For this review, take the finished solid that the model builds, in its own axes (mm). A direction names the side the tool comes from. Give positions to 0.01 mm unless a question says otherwise; leave off trailing zeros. Write each loop counter-clockwise with the first axis right and the second up, starting at its lowest first coordinate (ties: lowest second). Pieces come first, ordered by that corner, then holes. Notation, with made-up numbers: (53.5, 2.5) -> (60.5, 2.5) arc R11 ccw to (60.5, 9.5) -> close; hole circle Ø5 at (67, 31). An arc over 180 degrees is marked (long way). Answer as CSV lines item,"result".
```python
from build123d import *

# Parameters (mm, degrees)
F0_W     = 60
F0_H     = 40
F0_R     = 1
F1_DEPTH = 2
F2_W     = 8.5
F2_H     = 19
F3_DEPTH = 4
F4_W     = 34
F4_H     = 19
F5_DEPTH = 7
F6_W     = 2.5
F6_H     = 15
F6_W_2   = 6.5
F7_DEPTH = 4.3


with BuildPart() as f1:
    # F0 (on Front) → F1 (new body)
    with BuildSketch(Plane.XZ):
        Rectangle(F0_W, F0_H)
        with Locations((-28, -18)):
            Circle(F0_R, mode=Mode.SUBTRACT)
        with Locations((28, -18)):
            Circle(F0_R, mode=Mode.SUBTRACT)
        with Locations((-28, 18)):
            Circle(F0_R, mode=Mode.SUBTRACT)
        with Locations((28, 18)):
            Circle(F0_R, mode=Mode.SUBTRACT)
    extrude(amount=F1_DEPTH)

    # F2 (on face) → F3 (join)
    with BuildSketch(Plane(origin=(0, 0, 0), x_dir=(-1, 0, 0), z_dir=(0, 1, 0))):
        with Locations((20.25, 4.5)):
            Rectangle(F2_W, F2_H)
    extrude(amount=F3_DEPTH)

    # F4 (on face) → F5 (join)
    with BuildSketch(Plane(origin=(0, 0, 0), x_dir=(-1, 0, 0), z_dir=(0, 1, 0))):
        with Locations((-6.5, 3.5)):
            Rectangle(F4_W, F4_H)
    extrude(amount=F5_DEPTH)

    # F6 (on face) → F7 (join)
    with BuildSketch(Plane(origin=(0, 7, 0), x_dir=(-1, 0, 0), z_dir=(0, 1, 0))):
        with Locations((-22.25, 3.5)):
            Rectangle(F6_W, F6_H)
        with Locations((-26.75, 3.5)):
            Rectangle(F6_W_2, F6_H)
    extrude(amount=F7_DEPTH)


solid = f1.part
```
Q1. Add section C-C (z = 18). Write out the cut boundary in (x, y).
Answer block:
outline,"(-30, -2) -> (-29, -2) -> (-29, 0) -> (-30, 0) -> close; (-27, -2) -> (27, -2) -> (27, 0) -> (-27, 0) -> close; (29, -2) -> (30, -2) -> (30, 0) -> (29, 0) -> close"
Q2. Add section A-A (x = 28). Write out the cut boundary in (y, z).
Answer block:
outline,"(-2, -20) -> (0, -20) -> (0, -19) -> (-2, -19) -> close; (-2, -17) -> (0, -17) -> (0, 17) -> (-2, 17) -> close; (-2, 19) -> (0, 19) -> (0, 20) -> (-2, 20) -> close; (7, -4) -> (11.3, -4) -> (11.3, 11) -> (7, 11) -> close"
Q3. Clearance check with flat-ended pins moving along their axes: pin 1 (3.5 mm diameter, centred on x = 7.5, y = 2.5, fed in from +Z); pin 2 (4.5 mm diameter, centred on x = 27.5, y = 9.5, fed in from -Z); pin 3 (2.5 mm diameter, centred on x = 28, z = -18, fed in from +Y). State where each tip first meets the part, or that it passes through.
Answer block:
pin 1,"stops at z = 13"
pin 2,"stops at z = -4"
pin 3,"stops at y = 0"
Q4. Add section D-D (x = -5.5). Write out the cut boundary in (y, z), plus the area to 3 significant figures.
Answer block:
outline,"(-2, -20) -> (0, -20) -> (0, -6) -> (7, -6) -> (7, 13) -> (0, 13) -> (0, 20) -> (-2, 20) -> close"
area,"213 mm2"
Q5. To check wall thickness, follow probe 1 along Z at (x, y) = (-28, -1.35); probe 2 along X at (y, z) = (2.5, -2.5); probe 3 along Y at (x, z) = (13, 2). State the ranges of each line that lie inside material, in increasing order. Write a range as [from, to].
Answer block:
probe 1,"z = [-20, -19], [-17, 17], [19, 20]"
probe 2,"x = [-24.5, -16], [-10.5, 23.5]"
probe 3,"y = [-2, 7]"
Q6. Draft analysis for pull direction Z (two halves, no side actions). For faces 1 (the flat face through (-24.5, 2, 4)), 2 (the cylindrical face through (-28, -1, 17)), 3 (the flat face through (26, 9, -4)), state which applies: released by +Z, released by -Z, zero draft, split by the parting line, or undercut.
Answer block:
face 1,"zero draft"
face 2,"undercut"
face 3,"released by -Z"
Q7. Add section B-B (y = 3.25). Write out the cut boundary in (x, z).
Answer block:
outline,"(-24.5, -5) -> (-16, -5) -> (-16, 14) -> (-24.5, 14) -> close; (-10.5, -6) -> (23.5, -6) -> (23.5, 13) -> (-10.5, 13) -> close"
Q8. For faces 4 (the flat face through (23.5, 3, 3)), 5 (the flat face through (-20, 2, 14)), 6 (the flat face through (7, 3, 13)), 7 (the flat face through (-16, 2, 4)), list the 3-axis set-ups (+Z, -Z, +X, -X, +Y, -Y) from which the entire face can be reached by the end or side of a thin tool; tool diameter is ignored.
Answer block:
face 4,"+Z, -Z, +X"
face 5,"+Z, +X, -X, +Y"
face 6,"+Z, +X, +Y"
face 7,"+Z, -Z, +Y"
